Autodesk Inventor part; units mm, degrees
ref_plane "YZ Plane" through (0, 0, 0) normal (1, 0, 0) x (0, 1, 0)
ref_plane "XZ Plane" through (0, 0, 0) normal (0, 1, 0) x (-1, 0, 0)
ref_plane "XY Plane" through (0, 0, 0) normal (0, 0, 1) x (1, 0, 0)
sketch "Sketch1" plane through (0, 0, 0) normal (0, 0, 1) x (1, 0, 0)
  circle A0 centre (0, 0) radius 15
  arc A1 (15, -20) -> (-15, -20) centre (0, 0) ccw
  line L0 (-15, -20) -> (-15, -35)
  line L1 (-15, -35) -> (15, -35)
  line L2 (15, -20) -> (15, -35)
  dimension "d0" = 30
  dimension "d1" = 50
  dimension "d2" = 15
extrude "Extrusion1" add sketch "Sketch1" along normal blind 20
sketch "Sketch2" plane through (0, 0, 20) normal (0, 0, 1) x (1, 0, 0)
  point P0 (0, 0)
  point P1 (-19.9785, -0.185)
  point P2 (20.4097, 0.2462)
hole "Hole1" at (0, 0, 20) at (-19.9785, -0.185, 20) at (20.4097, 0.2462, 20) direction (0, 0, -1) diameter 5 end through all
fillet "Fillet1" radius 6 2 edges at (15, -20, 10) (-15, -20, 10)
properties part number "TPS base"
Design review of the part built by this model. Coordinates are the model's own, in mm. A direction names the side the tool comes from. Give positions to 0.01 mm unless a question says otherwise; leave off trailing zeros. Loops run counter-clockwise (first coordinate to the right, second up) from the corner with the lowest first, then second, coordinate; pieces in that order, holes last. Notation, with made-up numbers: (14, 84) - (50, 84) arc R9 cw to (50, 96) - close; hole circle Ø9 at (-32, 12). An arc over 180 degrees is marked (long way). Write item = value, one per line.
1) Draft analysis for pull direction X (two halves, no side actions). For faces 1 (the face through (-22.457, 0.14, 9.86)), 2 (the face through (-11, -11, 20)), 3 (the face through (15, -29, 10)), state which applies: +X half, -X half, draft (parallel to the pull), parting line (faces both ways), or undercut.
Result sheet:
face_1 = undercut
face_2 = draft
face_3 = +X half
2) Take a section at D-D on z = 6.5. State the section outline as (x, y) points (1 decimal), and give its area (3 significant figures).
Result sheet:
outline = (-16.9, -18.4) arc R6 cw to (-15, -22.8) - (-15, -35) - (15, -35) - (15, -22.8) arc R6 cw to (16.9, -18.4) arc R25 ccw (long way) to start; hole circle Ø5 at (-20, -0.2); hole circle Ø30 at (0, 0); hole circle Ø5 at (20.4, 0.2)
area = 1,570 mm2
3) Clearance check with flat-ended pins moving along their axes: pin 1 Ø3 at (y, z) = (-28, 14.5) entering from +X; pin 2 Ø1.5 at (x, z) = (18.5, 17) entering from -Y; pin 3 Ø8 at (x, z) = (6, 7.5) entering from +Y; pin 4 Ø24 at (x, y) = (0, 0) entering from +Z. State where each tip first meets the part, or that it passes through.
Result sheet:
pin_1 = 15
pin_2 = -17.61
pin_3 = 24.92
pin_4 = through
4) Take a section at A-A on x = 0. State the section outline as (y, z) points, and give its area (3 significant figures).
Result sheet:
outline = (-35, 0) - (-15, 0) - (-15, 20) - (-35, 20) - close; (15, 0) - (25, 0) - (25, 20) - (15, 20) - close
area = 600 mm2
5) Take a section at C-C on y = 0. State the section outline as (x, z) points.
Result sheet:
outline = (-25, 0) - (-22.47, 0) - (-22.47, 20) - (-25, 20) - close; (-17.49, 0) - (-15, 0) - (-15, 20) - (-17.49, 20) - close; (15, 0) - (17.92, 0) - (17.92, 20) - (15, 20) - close; (22.9, 0) - (25, 0) - (25, 20) - (22.9, 20) - close
6) Take a section at B-B on y = -8. State the section outline as (x, z) points.
Result sheet:
outline = (-23.69, 0) - (-12.69, 0) - (-12.69, 20) - (-23.69, 20) - close; (12.69, 0) - (23.69, 0) - (23.69, 20) - (12.69, 20) - close
7) To check wall thickness, follow line 1 (X direction, y = -25, z = 10.5); line 2 (Y direction, x = -20, z = 8.5); line 3 (X direction, y = 3, z = 14.5). State the ranges of each line that lie inside material, in increasing order.
Result sheet:
line_1 = -15 to 15
line_2 = -15 to -2.68, 2.31 to 15
line_3 = -24.82 to -14.7, 14.7 to 24.82
8) Tool access review of faces 4 (the face through (0, -35, 10)), 5 (the face through (-15, -29, 10)): name each direction out of +Z, -Z, +X, -X, +Y, -Y from which nothing blocks a thin tool from reaching the whole face with its end or side.
Result sheet:
face_4 = +Z, -Z, +X, -X, -Y
face_5 = +Z, -Z, -X, -Y
